from build123d import *

# Parameters (mm, degrees)
CROQUIS1_R              = 7.5
SALIENTE_EXTRUIR1_DEPTH = 10
CROQUIS2_W              = 25
CROQUIS2_H              = 8
SALIENTE_EXTRUIR2_DEPTH = 10


with BuildPart() as part:
    # Croquis1 → Saliente-Extruir1 (new body)
    with BuildSketch(Plane(origin=(0, 0, 0), x_dir=(0, 0, -1), z_dir=(1, 0, 0))):
        with BuildLine():
            Line((0, 0), (-25, 0))
            Line((-25, 0), (-25, 17.5))
            ThreePointArc((-25, 17.5), (-12.5, 30), (0, 17.5))
            Line((0, 17.5), (0, 0))
        make_face()
        with Locations((-12.5, 17.5)):
            Circle(CROQUIS1_R, mode=Mode.SUBTRACT)
    extrude(amount=SALIENTE_EXTRUIR1_DEPTH)

    # Croquis2 → Saliente-Extruir2 (add)
    with BuildSketch(Plane(origin=(10, 0, 0), x_dir=(0, 0, -1), z_dir=(1, 0, 0))):
        with Locations((-12.5, 4)):
            Rectangle(CROQUIS2_W, CROQUIS2_H)
    extrude(amount=SALIENTE_EXTRUIR2_DEPTH)


solid = part.part
Verification items for the finished model (mm, model axes). A direction names the side the tool comes from. Round coordinates to 2 decimals unless told otherwise and drop trailing zeros. Order: outer loops, then holes, each group sorted by start corner. A loop starts at its lowest first (then second) coordinate and runs counter-clockwise, first axis right, second up.
1. Release check for a two-part mould opening along Z. For faces 3 (the cylindrical face through (4.9, 22.6, 18)), 4 (the flat face through (8, 7, 25)), 5 (the flat face through (20, 4, 13)), 6 (the flat face through (8, 7, 0)) record: +Z half, -Z half, draft (parallel to the pull), parting line (faces both ways), or undercut.
Final values:
face 3: undercut
face 4: +Z half
face 5: draft
face 6: -Z half
2. Section check D-D on z = 5.5. Record the cut outline in (x, y).
Final values:
outline: (0, 0) - (20, 0) - (20, 8) - (10, 8) - (10, 14.81) - (0, 14.81) - close; (0, 20.19) - (10, 20.19) - (10, 27.86) - (0, 27.86) - close
3. Section check C-C on x = 6. Record the cut outline in (y, z), then the cut area to 3 significant figures.
Final values:
outline: (0, 0) - (17.5, 0) arc R12.5 ccw to (17.5, 25) - (0, 25) - close; hole circle Ø15 at (17.5, 12.5)
area: 506 mm2
4. Section check A-A on y = 22. Record the cut outline in (x, z), then the cut area to 3 significant figures.
Final values:
outline: (0, 0.84) - (10, 0.84) - (10, 6.5) - (0, 6.5) - close; (0, 18.5) - (10, 18.5) - (10, 24.16) - (0, 24.16) - close
area: 113 mm2
5. Go/stop test with flat-tipped pins: P1, Ø4, axis at x = 10, z = 15, coming from the +Y side; P2, Ø8, axis at x = 17, z = 9.5, coming from the +Y side. Record where each tip stops, or that it passes through.
Final values:
P1: stops at y = 29.99
P2: stops at y = 8
6. Section check B-B on z = 12.5. Record the cut outline in (x, y).
Final values:
outline: (0, 0) - (20, 0) - (20, 8) - (10, 8) - (10, 10) - (0, 10) - close; (0, 25) - (10, 25) - (10, 30) - (0, 30) - close
7. Thickness scan on L1, parallel to Y at x = 8.25, z = 12.5; L2, parallel to Y at x = 9.75, z = 2.5; L3, parallel to X at y = 28.5, z = 11.5. Record the ranges inside material, lowest first.
Final values:
L1: y = 0 to 10, 25 to 30
L2: y = 0 to 25
L3: x = 0 to 10
8. Access from +Z, -Z, +X, -X, +Y, -Y to the whole of each face (thin tool, end or side, straight path). Record for faces 1 (the flat face through (10, 24, 18)), 2 (the flat face through (10, 0, 13)).
Final values:
face 1: +Z, -Z, +X, +Y
face 2: +Z, -Z, +X, -X, -Y
